Here's how the part is built. I have some questions about the finished solid (model axes, mm). Face numbers are marked on the shaded views. A direction names the side the tool comes from. Coordinates: 2 decimals unless noted, no trailing zeros. Write each loop counter-clockwise with the first axis right and the second up, starting at its lowest first coordinate (ties: lowest second). Pieces come first, ordered by that corner, then holes. Notation, with made-up numbers: (87, -39.75) -> (92, -39.75) arc R17 cw to (92, -29.75) -> close; hole circle Ø8 at (73.5, 64.25). An arc over 180 degrees is marked (long way). Use a Markdown table: item, result. Add a question column.
Autodesk Inventor part; units mm, degrees
ref_plane "YZ Plane" through (0, 0, 0) normal (1, 0, 0) x (0, 1, 0)
ref_plane "XZ Plane" through (0, 0, 0) normal (0, 1, 0) x (-1, 0, 0)
ref_plane "XY Plane" through (0, 0, 0) normal (0, 0, 1) x (1, 0, 0)
sketch "Sketch1" plane through (0, 0, 0) normal (0, 1, 0) x (-1, 0, 0)
  line L0 (25, 22.5) -> (-25, 22.5)
  line L1 (-25, 22.5) -> (-25, -100)
  line L2 (-25, -100) -> (25, -100)
  line L3 (25, -100) -> (25, 22.5)
  circle A0 centre (0, 0) radius 4
  dimension "d0" = 50
  dimension "d1" = 22.5
  dimension "d2" = 25
  dimension "d3" = 122.5
  dimension "d4" = 8
extrude "Extrusion1" add sketch "Sketch1" along normal blind 5
sketch "Sketch2" plane through (0, 5, 0) normal (0, 1, 0) x (1, 0, 0)
  line L0 (-25, 100) -> (-25, -22.5)
  line L1 (25, -22.5) -> (25, 100)
  line L2 (-25, -22.5) -> (25, -22.5)
  line L3 (25, -22.5) -> (25, 100)
  line L4 (25, 100) -> (-25, 100)
  line L5 (-25, 100) -> (-25, -22.5)
  line L6 (-20, -17.5) -> (20, -17.5)
  line L7 (20, -17.5) -> (20, 95)
  line L8 (20, 95) -> (-20, 95)
  line L9 (-20, 95) -> (-20, -17.5)
  point P0 (0, 0)
  dimension "d7" = 5
  dimension "d8" = 5
  dimension "d9" = 5
  dimension "d10" = 5
extrude "Extrusion2" add sketch "Sketch2" along normal blind 50
sketch "Sketch3" plane through (0, 5, 0) normal (0, 1, 0) x (1, 0, 0)
  line L0 (-20, 95) -> (-20, -17.5)
  line L1 (20, -17.5) -> (20, 95)
  line L2 (-20, -17.5) -> (20, -17.5)
  line L3 (20, -17.5) -> (20, 14.5)
  line L4 (20, 14.5) -> (-20, 14.5)
  line L5 (-20, 14.5) -> (-20, -17.5)
  point P0 (0, 0)
  dimension "d13" = 32
extrude "Extrusion3" add sketch "Sketch3" along normal blind 30
sketch "Sketch4" plane through (25, 0, -100) normal (0, 0, -1) x (-1, 0, 0)
  circle A0 centre (25, 22.5) radius 6.5
  line L0 (0, 0) -> (50, 0)
  line L1 (50, 0) -> (50, 55)
  circle A1 centre (25, 29.5) radius 15.5
  line L2 (25, 29.5) -> (45.4383, 29.5)
  line L3 (45.4383, 29.5) -> (2.3057, 29.5)
  line L4 (25, 29.5) -> (33.9734, 13.9576)
  line L5 (25, 29.5) -> (15.8246, 13.6078)
  line L6 (25, 29.5) -> (33.427, 44.096)
  line L7 (25, 29.5) -> (15.5571, 45.8556)
  circle A2 centre (40.5, 29.5) radius 1.5
  circle A3 centre (32.75, 42.9234) radius 1.5
  circle A4 centre (17.25, 42.9234) radius 1.5
  circle A5 centre (9.5, 29.5) radius 1.5
  circle A6 centre (17.25, 16.0766) radius 1.5
  circle A7 centre (32.75, 16.0766) radius 1.5
  point P0 (25, 0)
  dimension "d16" = 22.5
  dimension "d17" = 13
  dimension "d18" = 25
  dimension "d19" = 7
  dimension "d20" = 31
  dimension "d21" = 60
  dimension "d22" = 60
  dimension "d23" = 60
  dimension "d24" = 60
  dimension "d25" = 25
  dimension "d26" = 3
  dimension "d27" = 3
  dimension "d28" = 3
  dimension "d29" = 3
  dimension "d30" = 3
  dimension "d31" = 3
extrude "Extrusion4" cut sketch "Sketch4" against normal blind 30 contours A0 L4 | L4 A0 L5 | L5 A0 | A7 A1 L4 | L4 A1 A7 | A2 A1 L2 | L2 A1 A2 | A5 A1 L3 | L3 A1 A5 | A3 A1 L6 | L6 A1 A3 | A4 A1 L7 | L7 A1 A4 | A6 A1 L5 | L5 A1 A6 | L4 A7 A1 | A1 A7 L4 | L2 A2 A1 | A1 A2 L2 | L3 A5 A1 | A1 A5 L3 | A1 A3 | L7 A4 A1 | A1 A4 L7 | L5 A6 A1 | A1 A6 L5 picked at (24.9025, 21.8029)
sketch "Sketch5" plane through (0, 0, 0) normal (0, -1, 0) x (1, 0, 0)
  circle A0 centre (0, 0) radius 4
  circle A1 centre (0, 0) radius 9.5
  dimension "d34" = 19
extrude "Extrusion5" cut sketch "Sketch5" against normal blind 12.5 contours A0 | A1
sketch "Sketch6" plane through (0, 0, 0) normal (0, -1, 0) x (1, 0, 0)
  circle A0 centre (0, 0) radius 9.5
  circle A1 centre (0, 0) radius 11.5
  dimension "d37" = 23
extrude "Extrusion6" cut sketch "Sketch6" against normal blind 6.5 contours A0 | A1
sketch "Sketch7" plane through (0, 12.5, 0) normal (0, -1, 0) x (1, 0, 0)
  circle A0 centre (0, 0) radius 9.5
  circle A1 centre (0, 0) radius 6.2
  line L0 (0, 0) -> (0, 7.2993)
  line L1 (0, 0) -> (-6.3974, -3.6935)
  line L2 (0, 0) -> (6.4992, -3.7523)
  circle A2 centre (5.3694, -3.1) radius 1.45
  circle A3 centre (-5.3694, -3.1) radius 1.45
  circle A4 centre (0, 6.2) radius 1.45
  dimension "d40" = 12.4
  dimension "d41" = 120
  dimension "d42" = 120
  dimension "d43" = 2.9
  dimension "d44" = 2.9
  dimension "d45" = 2.9
extrude "Extrusion7" cut sketch "Sketch7" against normal blind 30 contours A4 L0 A1 | A1 A4 | A2 A1 | A1 L2 A2 | L0 A4 A1 | A1 A2 L2 | A3 L1 A1 | A1 A3 | A3 A1 L1
fillet "Fillet1" radius 3 4 edges at (20, 20, -14.5) (-20, 20, -14.5) (25, 27.5, 22.5) (-25, 27.5, 22.5)
sketch "Sketch8" plane through (0, 35, 0) normal (0, 1, 0) x (1, 0, 0)
  circle A0 centre (-5.3694, 3.1) radius 1.45
  circle A1 centre (-5.3694, 3.1) radius 4
  circle A2 centre (5.3694, 3.1) radius 1.45
  circle A3 centre (5.3694, 3.1) radius 4
  circle A4 centre (0, -6.2) radius 1.45
  circle A5 centre (0, -6.2) radius 4
  point P0 (0, 0)
  dimension "d49" = 8
  dimension "d50" = 8
  dimension "d51" = 8
extrude "Extrusion8" cut sketch "Sketch8" against normal blind 7
properties part number "Link3_v2"
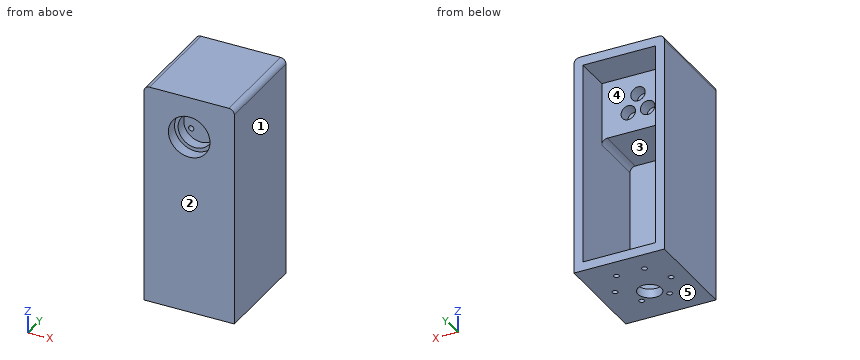
Q1. Which directions (+Z, -Z, +X, -X, +Y, -Y) give clear straight access to the entire face, cutting with the end or side of a thin tool? Please do the marked faces 4 and 5.
Q2. Thinking about a two-plate mould opening in X: for the marked faces 1, 2 and 3, which applies, released by +X, released by -X, zero draft, split by the parting line, or undercut?
Q3. Suppose I cut it at B-B, the plane y = 8.5. Write out the boundary of the cut face in (x, z), and give its area (3 significant figures).
Q4. Suppose I cut it at D-D, the plane y = 24. Write out the boundary of the cut face in (x, z), and give its area (3 significant figures).
Q5. Suppose I cut it at A-A, the plane x = 0. State how many separate pieces and enclosed holes the cut face has, and give its area (3 significant figures).
Q6. Suppose I cut it at C-C, the plane z = 6.2. Write out the boundary of the cut face in (x, y).
Q7. Please list where these lines run through material, in increasing order: line 1 (X direction, y = 23.25, z = -3.1); line 2 (Z direction, x = 0, y = 22.5); line 3 (X direction, y = 50, z = -87).
Q8. Will these pins go through, and if not, where does the flat tip stop? pin 1 (9 mm diameter, centred on x = -5.37, z = -3.1, fed in from -Y); pin 2 (4.5 mm diameter, centred on x = 5.37, z = -3.1, fed in from -Y); pin 3 (6 mm diameter, centred on x = 8.5, z = -32, fed in from -Y); pin 4 (6.5 mm diameter, centred on x = -1.5, z = 7.5, fed in from +Y).
Answer key:
| question | item | result |
|---|---|---|
| 1 | face 4 | +Y |
| 1 | face 5 | -Z, +X, -X, +Y, -Y |
| 2 | face 1 | released by +X |
| 2 | face 2 | zero draft |
| 2 | face 3 | undercut |
| 3 | outline | (-25, -100) -> (25, -100) -> (25, 19.5) arc R3 ccw to (22, 22.5) -> (-22, 22.5) arc R3 ccw to (-25, 19.5) -> close; hole (-20, -95) -> (20, -95) -> (20, -17.5) arc R3 ccw to (17, -14.5) -> (-17, -14.5) arc R3 ccw to (-20, -17.5) -> close; hole circle Ø19 at (0, 0) |
| 3 | area | 2,620 mm^2 |
| 4 | outline | (-25, -100) -> (-6.32, -100) -> (-6.32, -95) -> (-20, -95) -> (-20, -17.5) arc R3 cw to (-17, -14.5) -> (17, -14.5) arc R3 cw to (20, -17.5) -> (20, -95) -> (6.32, -95) -> (6.32, -100) -> (25, -100) -> (25, 19.5) arc R3 ccw to (22, 22.5) -> (-22, 22.5) arc R3 ccw to (-25, 19.5) -> close; hole circle Ø2.9 at (-5.37, -3.1); hole circle Ø2.9 at (0, 6.2); hole circle Ø2.9 at (5.37, -3.1) |
| 4 | area | 2,820 mm^2 |
| 5 | separate pieces | 3 |
| 5 | enclosed holes | 0 |
| 5 | area | 1,640 mm^2 |
| 6 | outline | (-25, 0) -> (-9.69, 0) -> (-9.69, 6.5) -> (-7.2, 6.5) -> (-7.2, 12.5) -> (-1.45, 12.5) -> (-1.45, 28) -> (-4, 28) -> (-4, 35) -> (-20, 35) -> (-20, 55) -> (-25, 55) -> close; (1.45, 12.5) -> (7.2, 12.5) -> (7.2, 6.5) -> (9.69, 6.5) -> (9.69, 0) -> (25, 0) -> (25, 55) -> (20, 55) -> (20, 35) -> (4, 35) -> (4, 28) -> (1.45, 28) -> close |
| 7 | line 1 | x = -25 to -6.82, -3.92 to 3.92, 6.82 to 25 |
| 7 | line 2 | z = -14.5 to 4.75, 7.65 to 22.5 |
| 7 | line 3 | x = -25 to -20, 20 to 25 |
| 8 | pin 1 | stops at y = 6.5 |
| 8 | pin 2 | stops at y = 12.5 |
| 8 | pin 3 | stops at y = 0 |
| 8 | pin 4 | stops at y = 35 |
